```python
from build123d import *

# Parameters (mm, degrees)
F1_DEPTH  = 32
F2_R      = 9.193205317
F4_DEPTH  = 11
F3_R      = 8.8221237906
F5_DEPTH  = 50.8
F6_R      = 16
F7_R      = 15.99999
F8_R      = 16
F9_R      = 15.99999
F10_R     = 10.6938119657
F11_DEPTH = 32


# Not quite as in the source:
# - a fillet or chamfer is up to 0.001 mm smaller than in the source, because OpenCascade refuses the exact size


with BuildPart() as f1:
    # F0 (on Top) → F1 (new body)
    with BuildSketch(Plane.XY):
        Polygon((16.5285665829, 19.762864985), (-24.4714334171, 19.762864985), (-24.4714334171, 8.762864985), (16.5285665829, 8.762864985), (16.5285665829, -9.237135015), (-24.4714334171, -9.237135015), (-24.4714334171, -20.237135015), (27.5285665829, -20.237135015), (27.5285665829, 19.762864985), align=None)
    extrude(amount=F1_DEPTH)

    # F2 (on face) → F4 (cut)
    with BuildSketch(Plane.XZ.offset(20.237135015)):
        with Locations((0, 14.8110119626)):
            Circle(F2_R)
    extrude(amount=-F4_DEPTH, mode=Mode.SUBTRACT)

    # F3 (on Front) → F5 (cut)
    with BuildSketch(Plane.XZ):
        with Locations((0, 15.7271567732)):
            Circle(F3_R)
    extrude(amount=-F5_DEPTH, mode=Mode.SUBTRACT)

    # F6
    f6_edges = [f1.edges().sort_by_distance(p)[0] for p in [
        (-24.471433, -14.737135, 32),
    ]]
    fillet(f6_edges, radius=F6_R)

    # F7 (radius 16 in the source; OpenCascade refuses exactly that, so slightly less here)
    f7_edges = [f1.edges().sort_by_distance(p)[0] for p in [
        (-24.471433, -14.737135, 0),
    ]]
    fillet(f7_edges, radius=F7_R)

    # F8
    f8_edges = [f1.edges().sort_by_distance(p)[0] for p in [
        (-24.471433, 14.262865, 32),
    ]]
    fillet(f8_edges, radius=F8_R)

    # F9 (radius 16 in the source; OpenCascade refuses exactly that, so slightly less here)
    f9_edges = [f1.edges().sort_by_distance(p)[0] for p in [
        (-24.471433, 14.262865, 0),
    ]]
    fillet(f9_edges, radius=F9_R)

    # F10 (on face) → F11 (join)
    with BuildSketch(Plane.YZ.offset(27.5285665829)):
        with Locations((0, 15.7271567732)):
            Circle(F10_R)
    extrude(amount=F11_DEPTH)


solid = f1.part
```
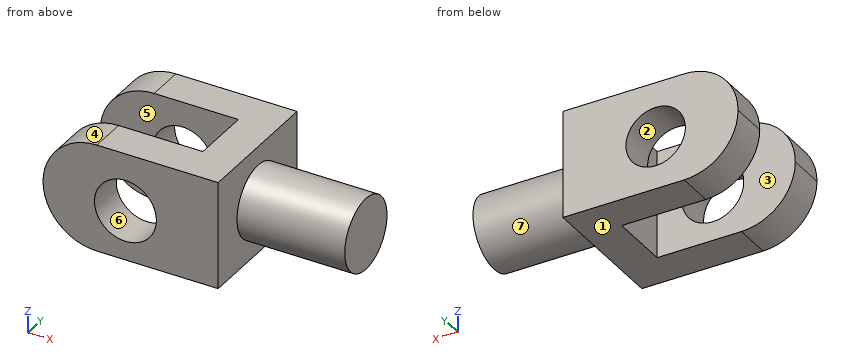
For this review, take the finished solid that the model builds, in its own axes (mm). Face numbers are marked on the shaded views. A direction names the side the tool comes from. Coordinates: 2 decimals unless noted, no trailing zeros. Write each loop counter-clockwise with the first axis right and the second up, starting at its lowest first coordinate (ties: lowest second). Pieces come first, ordered by that corner, then holes. Notation, with made-up numbers: (30.5, -12) - (87.5, -12) arc R12 cw to (87.5, -4) - close; hole circle Ø5 at (-8.5, 59). An arc over 180 degrees is marked (long way). Put each result on its own line as item: value.
1. Machinability: for the marked faces 4, 5, 6 and 7, which of the approach directions +Z, -Z, +X, -X, +Y, -Y give a long, thin tool a straight path to every point of the face, cutting with its end or side? Answer none if there is none.
Values found:
face 4: +Z, -X, +Y, -Y
face 5: +Z, -Z, -X
face 6: -Y
face 7: +X
2. For pin 1 (6 mm diameter, centred on x = 41, z = 14.5, fed in from -Y); pin 2 (5 mm diameter, centred on x = 36.5, y = 13.5, fed in from +Z); pin 3 (9 mm diameter, centred on y = -3, z = 9, fed in from -X); pin 4 (3 mm diameter, centred on y = 10.5, z = 27, fed in from +X), all flat-tipped, find the tip position at first contact; note any pin that passes through.
Values found:
pin 1: y = -10.69
pin 2: through
pin 3: x = 16.53
pin 4: x = 27.53
3. Add section A-A, the plane x = 0. Give the boundary of the cut face in (y, z), then the cut area to 3 significant figures.
Values found:
outline: (-20.24, 0) - (-9.24, 0) - (-9.24, 5.62) - (-20.24, 5.62) - close; (-20.24, 24) - (-9.24, 24) - (-9.24, 32) - (-20.24, 32) - close; (8.76, 0) - (19.76, 0) - (19.76, 6.91) - (8.76, 6.91) - close; (8.76, 24.55) - (19.76, 24.55) - (19.76, 32) - (8.76, 32) - close
area: 308 mm²
4. Add section B-B, the plane z = 14. Give the boundary of the cut face in (x, y).
Values found:
outline: (-24.35, -20.24) - (-9.16, -20.24) - (-9.16, -9.24) - (-24.35, -9.24) - close; (-24.35, 8.76) - (-8.65, 8.76) - (-8.65, 19.76) - (-24.35, 19.76) - close; (8.65, 8.76) - (16.53, 8.76) - (16.53, -9.24) - (9.16, -9.24) - (9.16, -20.24) - (27.53, -20.24) - (27.53, -10.55) - (59.53, -10.55) - (59.53, 10.55) - (27.53, 10.55) - (27.53, 19.76) - (8.65, 19.76) - close
5. Add section C-C, the plane y = 0. Give the boundary of the cut face in (x, z), then the cut area to 3 significant figures.
Values found:
outline: (16.53, 0) - (27.53, 0) - (27.53, 5.03) - (59.53, 5.03) - (59.53, 26.42) - (27.53, 26.42) - (27.53, 32) - (16.53, 32) - close
area: 1,040 mm²
6. Mouldability with a two-part tool opening along Z and no side actions: class the marked faces 1, 2 and 3 as released by +Z, released by -Z, zero draft, split by the parting line, or undercut.
Values found:
face 1: released by -Z
face 2: undercut
face 3: zero draft
7. Wall thickness on probe 1 along Y at (x, z) = (2, 4); probe 2 along Z at (x, y) = (0, 12.75); probe 3 along X at (y, z) = (3.5, 23): over which ranges is each line inside the solid? List them lowest first.
Values found:
probe 1: -20.24 to -9.24, 8.76 to 19.76
probe 2: 0 to 6.91, 24.55 to 32
probe 3: 16.53 to 59.53
